```python
from build123d import *

# Parameters (mm, degrees)
SKETCH1_W                = 57
SKETCH1_H                = 57
BOSS_EXTRUDE1_DEPTH      = 52
SKETCH2_R                = 3.175
BOSS_EXTRUDE2_DEPTH      = 21
FILLET1_R                = 2
SKETCH9_R                = 19.05
BOSS_EXTRUDE3_DEPTH      = 1.6
SKETCH11_R               = 2.75
CUT_EXTRUDE3_DEPTH       = 66.791336816
CUT_EXTRUDE2_START       = -15
CUT_EXTRUDE2_DEPTH       = 15
SKETCH12_W               = 9.86
SKETCH12_H               = 9.86
CUT_EXTRUDE4_DEPTH       = 47
FILLET2_R                = 2
CIRPATTERN1_COUNT        = 4
FILLET2_OF_CIRPATTERN1_R = 2


with BuildPart() as part:
    # Sketch1 → Boss-Extrude1 (new body)
    with BuildSketch(Plane.XY):
        Rectangle(SKETCH1_W, SKETCH1_H)
    extrude(amount=BOSS_EXTRUDE1_DEPTH)

    # Sketch2 → Boss-Extrude2 (add)
    with BuildSketch(Plane.XY.offset(52)):
        with Locations(Location((0, 0, 0), (0, 0, 180))):
            Circle(SKETCH2_R)
    extrude(amount=BOSS_EXTRUDE2_DEPTH)

    # Fillet1
    fillet1_edges = [part.edges().sort_by_distance(p)[0] for p in [
        (28.5, -28.5, 26),
        (-28.5, -28.5, 26),
        (-28.5, 28.5, 26),
        (28.5, 28.5, 26),
    ]]
    fillet(fillet1_edges, radius=FILLET1_R)

    # Sketch9 → Boss-Extrude3 (add)
    with BuildSketch(Plane.XY.offset(52)):
        with Locations(Location((0, 0, 0), (0, 0, 180))):
            Circle(SKETCH9_R)
    extrude(amount=BOSS_EXTRUDE3_DEPTH)

    # Sketch11 → Cut-Extrude3 (cut, through all)
    with BuildSketch(Plane.XY.offset(52)):
        with Locations((23.57, 23.57)):
            Circle(SKETCH11_R)
        with Locations((23.57, -23.57)):
            Circle(SKETCH11_R)
        with Locations((-23.57, -23.57)):
            Circle(SKETCH11_R)
        with Locations((-23.57, 23.57)):
            Circle(SKETCH11_R)
    extrude(amount=-CUT_EXTRUDE3_DEPTH, mode=Mode.SUBTRACT)

    # Sketch10 → Cut-Extrude2 (cut)
    with BuildSketch(Plane.XY.offset(73).offset(CUT_EXTRUDE2_START)):
        with BuildLine():
            Line((-1.710263138, 2.675), (1.710263138, 2.675))
            ThreePointArc((1.710263138, 2.675), (0, 3.175), (-1.710263138, 2.675))
        make_face()
    extrude(amount=CUT_EXTRUDE2_DEPTH, mode=Mode.SUBTRACT)

    # Sketch12 → Cut-Extrude4 (cut)
    with BuildSketch(Plane(origin=(0, 0, 0), x_dir=(-1, 0, 0), z_dir=(0, 0, -1))):
        with Locations((-23.57, 23.57)):
            Rectangle(SKETCH12_W, SKETCH12_H)
    cut_extrude4 = extrude(amount=-CUT_EXTRUDE4_DEPTH, mode=Mode.SUBTRACT)

    # Fillet2
    fillet2_edges = [part.edges().sort_by_distance(p)[0] for p in [
        (18.64, 18.64, 23.5),
    ]]
    fillet(fillet2_edges, radius=FILLET2_R)

    # CirPattern1: Cut-Extrude4 ×4 about axis
    cirpattern1_axis = Axis((0, 0, 0), (0, 0, 1))
    for i in range(1, CIRPATTERN1_COUNT):
        add(cut_extrude4.rotate(cirpattern1_axis, i * 360 / CIRPATTERN1_COUNT), mode=Mode.SUBTRACT)

    # Fillet2 of CirPattern1
    fillet2_of_cirpattern1_edges = [part.edges().sort_by_distance(p)[0] for p in [
        (-18.64, 18.64, 23.5),
        (-18.64, -18.64, 23.5),
        (18.64, -18.64, 23.5),
    ]]
    fillet(fillet2_of_cirpattern1_edges, radius=FILLET2_OF_CIRPATTERN1_R)


solid = part.part
```
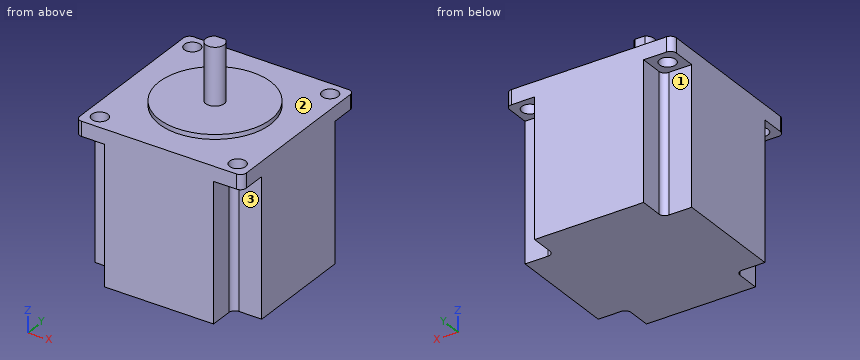
Here's how the part is built. I have some questions about the finished solid (model axes, mm). Face numbers are marked on the shaded views. A direction names the side the tool comes from. Coordinates: 2 decimals unless noted, no trailing zeros. Write each loop counter-clockwise with the first axis right and the second up, starting at its lowest first coordinate (ties: lowest second). Pieces come first, ordered by that corner, then holes. Notation, with made-up numbers: (8, 25.5) -> (15, 25.5) arc R17 cw to (15, 37.5) -> close; hole circle Ø11 at (23.25, -36). An arc over 180 degrees is marked (long way). Use a Markdown table: item, result. Add a question column.
(1) Please list where these lines run through material, in increasing order: line 1 (Y direction, x = -23.57, z = 49.3); line 2 (X direction, y = 23, z = 48); line 3 (Z direction, x = 13.5, y = -3.5).
(2) If we section it at C-C, the plane z = 48: Write out the boundary of the cut face in (x, y).
(3) If we section it at D-D, the plane x = 0: Write out the boundary of the cut face in (y, z) (3 decimals), and give its area (3 significant figures).
(4) I'm going to push flat-ended pins straight in: P1, Ø5, axis at x = -26, y = 23.5, coming from the -Z side; P2, Ø6.5, axis at x = -24.5, z = 13, coming from the +Y side; P3, Ø4, axis at x = -25, z = 28.5, coming from the -Y side; P4, Ø4.5, axis at x = 23.57, y = -23.57, coming from the -Z side. Where does each tip first touch, or does it pass through?
(5) If we section it at A-A, the plane x = 23.57: Write out the boundary of the cut face in (y, z), and give its area (3 significant figures).
(6) For the marked faces 1, 2 and 3, which set-ups out of +Z, -Z, +X, -X, +Y, -Y let a thin tool reach every point of the face, with its end or its side?
Outcome:
| question | item | result |
|---|---|---|
| 1 | line 1 | y = -28.5 to -26.32, -20.82 to 20.82, 26.32 to 28.5 |
| 1 | line 2 | x = -28.5 to -26.26, -20.88 to 20.88, 26.26 to 28.5 |
| 1 | line 3 | z = 0 to 53.6 |
| 2 | outline | (-28.5, -26.5) arc R2 ccw to (-26.5, -28.5) -> (26.5, -28.5) arc R2 ccw to (28.5, -26.5) -> (28.5, 26.5) arc R2 ccw to (26.5, 28.5) -> (-26.5, 28.5) arc R2 ccw to (-28.5, 26.5) -> close; hole circle Ø5.5 at (-23.57, -23.57); hole circle Ø5.5 at (-23.57, 23.57); hole circle Ø5.5 at (23.57, -23.57); hole circle Ø5.5 at (23.57, 23.57) |
| 3 | outline | (-28.5, 0) -> (28.5, 0) -> (28.5, 52) -> (19.05, 52) -> (19.05, 53.6) -> (3.175, 53.6) -> (3.175, 58) -> (2.675, 58) -> (2.675, 73) -> (-3.175, 73) -> (-3.175, 53.6) -> (-19.05, 53.6) -> (-19.05, 52) -> (-28.5, 52) -> close |
| 3 | area | 3,140 mm^2 |
| 4 | P1 | stops at z = 47 |
| 4 | P2 | stops at y = 18.64 |
| 4 | P3 | stops at y = -18.64 |
| 4 | P4 | passes through |
| 5 | outline | (-28.5, 47) -> (-26.32, 47) -> (-26.32, 52) -> (-28.5, 52) -> close; (-20.82, 47) -> (-18.64, 47) -> (-18.64, 0) -> (18.64, 0) -> (18.64, 47) -> (20.82, 47) -> (20.82, 52) -> (-20.82, 52) -> close; (26.32, 47) -> (28.5, 47) -> (28.5, 52) -> (26.32, 52) -> close |
| 5 | area | 1,980 mm^2 |
| 6 | face 1 | -Z, -X, +Y |
| 6 | face 2 | +Z |
| 6 | face 3 | -Z, +X, -Y |
